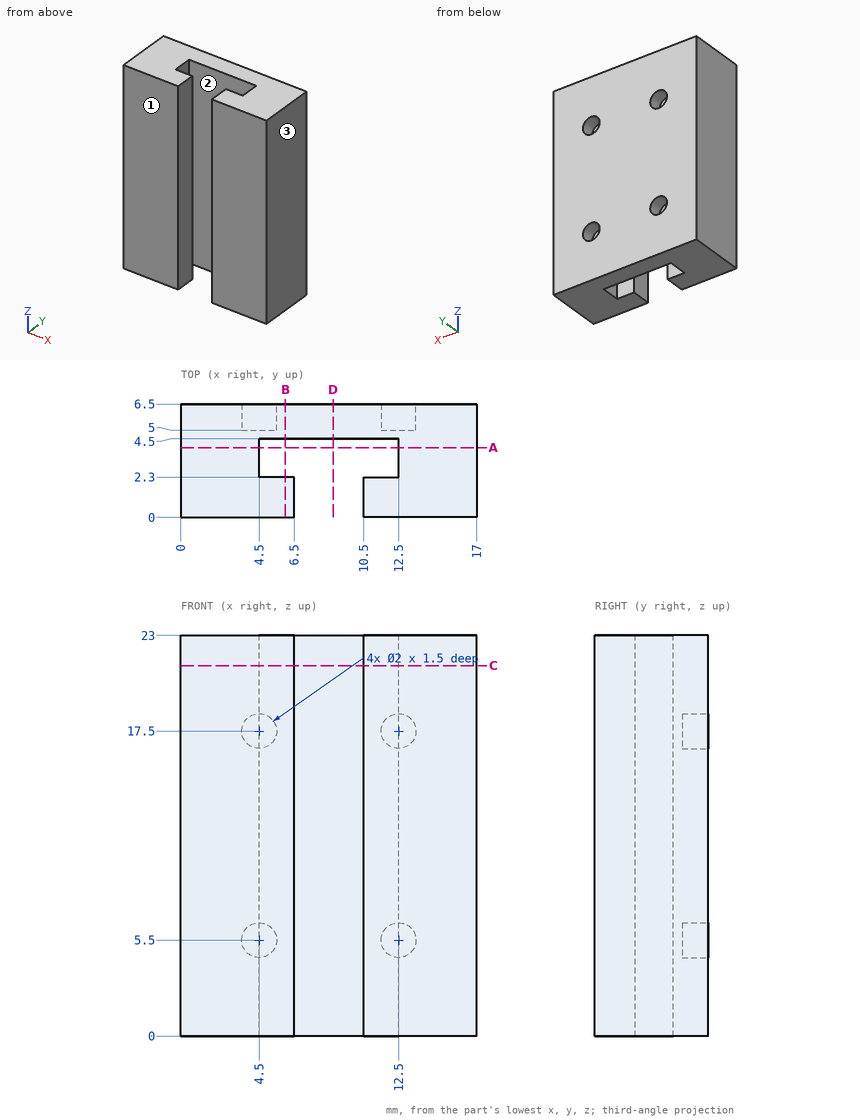
Geometry: see drawing. Coordinates: mm, zero at the bounding-box minimum. Give positions to 0.01 mm unless a question says otherwise; leave off trailing zeros. Loops run counter-clockwise (first coordinate to the right, second up) from the corner with the lowest first, then second, coordinate; pieces in that order, holes last. Notation, with made-up numbers: (31.5, 76) - (80.5, 76) arc R22 ccw to (80.5, 104) - close; hole circle Ø6 at (-25.75, 75.5). An arc over 180 degrees is marked (long way). Use CSV: the item, a comma, the result in double quotes. Start each with the question number.
1. Section C-C (z = 21.25). Output: boundary loops of the cut face in (x, y), then the cut area to 3 significant figures.
2. Draft query along Y for the marked faces 1, 2 and 3. Return one class per face: +Y half, -Y half, draft (parallel to the pull), parting line (faces both ways), or undercut.
3. Section B-B (x = 6). Output: boundary loops of the cut face in (y, z).
4. Section D-D (x = 8.75). Output: boundary loops of the cut face in (y, z), then the cut area to 3 significant figures.
5. Ray query, L1, parallel to Z at x = 12.5, y = 5.3; L2, parallel to X at y = 0.5, z = 15.5; L3, parallel to X at y = 3, z = 3.75. Return the intervals inside material, ascending.
6. Pin query (flat end, axial travel): pin 1 (1.8 mm diameter, centred on x = 4.5, z = 17.5, fed in from +Y); pin 2 (1 mm diameter, centred on x = 11.5, y = 3, fed in from -Z). Return the tip coordinate at first contact, or that it passes through.
7. Section A-A (y = 4). Output: boundary loops of the cut face in (x, z), then the cut area to 3 significant figures.
Response:
1,outline,"(0, 0) - (6.5, 0) - (6.5, 2.3) - (4.5, 2.3) - (4.5, 4.5) - (12.5, 4.5) - (12.5, 2.3) - (10.5, 2.3) - (10.5, 0) - (17, 0) - (17, 6.5) - (0, 6.5) - close"
1,area,"83.7 mm²"
2,face 1,"-Y half"
2,face 2,"undercut"
2,face 3,"draft"
3,outline,"(0, 0) - (2.3, 0) - (2.3, 23) - (0, 23) - close; (4.5, 0) - (6.5, 0) - (6.5, 23) - (4.5, 23) - close"
4,outline,"(4.5, 0) - (6.5, 0) - (6.5, 23) - (4.5, 23) - close"
4,area,"46.0 mm²"
5,L1,"0 to 4.5, 6.5 to 16.5, 18.5 to 23"
5,L2,"0 to 6.5, 10.5 to 17"
5,L3,"0 to 4.5, 12.5 to 17"
6,pin 1,"y = 5"
6,pin 2,"through"
7,outline,"(0, 0) - (4.5, 0) - (4.5, 23) - (0, 23) - close; (12.5, 0) - (17, 0) - (17, 23) - (12.5, 23) - close"
7,area,"207 mm²"
